from build123d import *

# Parameters (mm, degrees)
SALIENTE_EXTRUIR1_DEPTH = 6
REDONDEO1_R             = 0.3
REDONDEO2_R             = 1.2


with BuildPart() as part:
    # Croquis1 → Saliente-Extruir1 (new body)
    with BuildSketch(Plane.XY):
        with BuildLine():
            Line((0, 6.9), (120, 6.9))
            Line((120, 6.9), (120, 2.5))
            Line((120, 2.5), (126, 2.5))
            Line((126, 2.5), (126, 6.9))
            Line((126, 6.9), (370, 6.9))
            ThreePointArc((370, 6.9), (376.9, 0), (370, -6.9))
            Line((370, -6.9), (0, -6.9))
            ThreePointArc((0, -6.9), (-6.9, 0), (0, 6.9))
        make_face()
        with BuildLine():
            Line((0, 5.5), (118.6, 5.5))
            Line((118.6, 5.5), (118.6, 1.1))
            Line((118.6, 1.1), (127.4, 1.1))
            Line((127.4, 1.1), (127.4, 5.5))
            Line((127.4, 5.5), (370, 5.5))
            ThreePointArc((370, 5.5), (375.5, 0), (370, -5.5))
            Line((370, -5.5), (0, -5.5))
            ThreePointArc((0, -5.5), (-5.5, 0), (0, 5.5))
        make_face(mode=Mode.SUBTRACT)
    extrude(amount=SALIENTE_EXTRUIR1_DEPTH)

    # Redondeo1
    redondeo1_edges = [part.edges().sort_by_distance(p)[0] for p in [
        (120, 2.5, 3),
        (126, 2.5, 3),
        (127.4, 5.5, 3),
        (118.6, 5.5, 3),
    ]]
    fillet(redondeo1_edges, radius=REDONDEO1_R)

    # Redondeo2
    redondeo2_edges = [part.edges().sort_by_distance(p)[0] for p in [
        (120, 6.9, 3),
        (126, 6.9, 3),
        (127.4, 1.1, 3),
        (118.6, 1.1, 3),
    ]]
    fillet(redondeo2_edges, radius=REDONDEO2_R)


solid = part.part
Work out the finished part from the listing and answer in its coordinate system (mm). A direction names the side the tool comes from. Coordinates: 2 decimals unless noted, no trailing zeros. Order: outer loops, then holes, each group sorted by start corner. A loop starts at its lowest first (then second) coordinate and runs counter-clockwise, first axis right, second up. Notation, with made-up numbers: (73.25, 23.25) - (108.25, 23.25) arc R24 cw to (108.25, 50.25) - close; hole circle Ø9 at (40.5, 32.25). An arc over 180 degrees is marked (long way). Put each result on its own line as item: value. Start each with the question number.
1) Find section B-B (x = 64.5). Give the vertices of the cut face in (y, z).
2) For a pull along Y with two mould halves and no side action, classify faces 1 (the flat face through (123, 1.1, 3)), 2 (the flat face through (186, 6, 6)), 3 (the cylindrical face through (-6.9, -0.15, 2.96)) as released by +Y, released by -Y, zero draft, split by the parting line, or undercut.
3) For faces 4 (the flat face through (186, 6, 0)), 5 (the cylindrical face through (-5.5, -0.1, 3)), determine the directions among +Z, -Z, +X, -X, +Y, -Y from which every point of the face is accessible in a straight line to the end or side of a thin tool.
4) Flat-ended cylindrical pins translate along their axes: pin 1 (1.5 mm diameter, centred on y = 4, z = 4.5, fed in from +X); pin 2 (2.5 mm diameter, centred on y = 3, z = 3, fed in from +X); pin 3 (3 mm diameter, centred on y = 3, z = 4, fed in from -X) (3 decimals). Find the tip coordinate at first contact, or state that the pin passes through.
5) Find section C-C (y = -1.75). Give the vertices of the cut face in (x, z), plus the area to 3 significant figures.
6) Find the intervals of material crossed by line 1 (Y direction, x = 142.5, z = 4.9); line 2 (X direction, y = 4.5, z = 3.5); line 3 (X direction, y = 3.5, z = 1.15), in increasing order. Write a range as from..to.
7) Find section A-A (z = 2.1). Give the vertices of the cut face in (x, y).
Results list:
1. outline: (-6.9, 0) - (-5.5, 0) - (-5.5, 6) - (-6.9, 6) - close; (5.5, 0) - (6.9, 0) - (6.9, 6) - (5.5, 6) - close
2. face 1: undercut
2. face 2: zero draft
2. face 3: split by the parting line
3. face 4: -Z, +X, -X, +Y, -Y
3. face 5: +Z, -Z
4. pin 1: stops at x = 376.09
4. pin 2: stops at x = 376.67
4. pin 3: stops at x = -6.735
5. outline: (-6.67, 0) - (-5.21, 0) - (-5.21, 6) - (-6.67, 6) - close; (375.21, 0) - (376.67, 0) - (376.67, 6) - (375.21, 6) - close
5. area: 17.5 mm^2
6. line 1: y = -6.9..-5.5, 5.5..6.9
6. line 2: x = -5.23..-3.16, 118.6..120, 126..127.4, 373.16..375.23
6. line 3: x = -5.95..-4.24, 118.6..120, 126..127.4, 374.24..375.95
7. outline: (0, -6.9) - (370, -6.9) arc R6.9 ccw to (370, 6.9) - (127.2, 6.9) arc R1.2 ccw to (126, 5.7) - (126, 2.8) arc R0.3 cw to (125.7, 2.5) - (120.3, 2.5) arc R0.3 cw to (120, 2.8) - (120, 5.7) arc R1.2 ccw to (118.8, 6.9) - (0, 6.9) arc R6.9 ccw to start; hole (0, -5.5) - (370, -5.5) arc R5.5 ccw to (370, 5.5) - (127.7, 5.5) arc R0.3 ccw to (127.4, 5.2) - (127.4, 2.3) arc R1.2 cw to (126.2, 1.1) - (119.8, 1.1) arc R1.2 cw to (118.6, 2.3) - (118.6, 5.2) arc R0.3 ccw to (118.3, 5.5) - (0, 5.5) arc R5.5 ccw to start
